Input: part model. Units: mm. Frame: model coordinates. Face numbers are marked on the shaded views. A direction names the side the tool comes from. Round coordinates to 2 decimals unless told otherwise and drop trailing zeros. Loops run counter-clockwise (first coordinate to the right, second up) from the corner with the lowest first, then second, coordinate; pieces in that order, holes last. Notation, with made-up numbers: (82, 65.25) - (112, 65.25) arc R6 cw to (112, 74.25) - close; hole circle Ø1 at (36.5, 53). An arc over 180 degrees is marked (long way). Use CSV: the item, a comma, the result in double quotes. Start each with the question number.
1. Cut plane A-A (y = -1.5). Return loops of the section in (x, z).
2. Cut plane B-B (x = 20). Return loops of the section in (y, z).
3. Access query for the marked faces 1 and 2. Directions: +Z, -Z, +X, -X, +Y, -Y. A direction counts if a zero-diameter tool reaches every point of the face in a straight line with its end or side. Return the directions, or none.
4. Cut plane C-C (y = -30). Return loops of the section in (x, z), and give its area (3 significant figures).
5. Pull-direction query (Y, two-part tool) for the marked faces 3, 4 and 5; classes: +Y half, -Y half, draft (parallel to the pull), parting line (faces both ways), or undercut.
6. Cut plane D-D (x = 6). Return loops of the section in (y, z).
7. Pin query (flat end, axial travel): P1, Ø0.6, axis at x = 4.5, y = 0.5, coming from the +Z side; P2, Ø0.6, axis at y = 0.5, z = 10, coming from the -X side; P3, Ø5.5, axis at y = -20, z = 10, coming from the +X side. Return the tip coordinate at first contact, or that it passes through.
8. Material intervals for probe 1 along Z at (x, y) = (2.1, -20); probe 2 along X at (y, z) = (-2.15, 10); probe 3 along Y at (x, z) = (0.9, 10), sorted ascending. Write a range as from..to.
```python
from build123d import *

# Parameters (mm, degrees)
BOSS_EXTRUDE1_DEPTH = 3.5
BOSS_EXTRUDE2_DEPTH = 16.5
SKETCH4_R           = 2.2
CUT_EXTRUDE1_DEPTH  = 53.773099208
SKETCH5_R           = 2.2
CUT_EXTRUDE2_DEPTH  = 53.773099208
BOSS_EXTRUDE5_DEPTH = 36
SKETCH7_W           = 15
SKETCH7_H           = 1.1
CUT_EXTRUDE3_DEPTH  = 53.496095093
BOSS_EXTRUDE6_REACH = 57.429
SKETCH9_W           = 1.1
SKETCH9_H           = 15
CUT_EXTRUDE4_DEPTH  = 53.496095093
BOSS_EXTRUDE7_DEPTH = 3.5
SKETCH11_R          = 1.6
CUT_EXTRUDE5_DEPTH  = 54.518688325


with BuildPart() as part:
    # Sketch1 → Boss-Extrude1 (new body)
    with BuildSketch(Plane.XY):
        Polygon((0, -36), (0, 0), (36, 0), (36, -3), (3, -36), align=None)
    extrude(amount=BOSS_EXTRUDE1_DEPTH)

    # Sketch2 → Boss-Extrude2 (add)
    with BuildSketch(Plane.XY.offset(3.5)):
        Polygon((0, -36), (0, 0), (36, 0), (36, -3), (3, -3), (3, -36), align=None)
    extrude(amount=BOSS_EXTRUDE2_DEPTH)

    # Sketch4 → Cut-Extrude1 (cut, through all)
    with BuildSketch(Plane.XZ.offset(3)):
        with Locations(Location((20, 10, 0), (0, 0, 270))):
            Circle(SKETCH4_R)
    extrude(amount=-CUT_EXTRUDE1_DEPTH, mode=Mode.SUBTRACT)

    # Sketch5 → Cut-Extrude2 (cut, through all)
    with BuildSketch(Plane(origin=(3, 0, 0), x_dir=(0, 0, -1), z_dir=(1, 0, 0))):
        with Locations((-10, -20)):
            Circle(SKETCH5_R)
    extrude(amount=-CUT_EXTRUDE2_DEPTH, mode=Mode.SUBTRACT)

    # Sketch6 → Boss-Extrude5 (add, through all)
    with BuildSketch(Plane(origin=(36, 0, 0), x_dir=(0, 0, -1), z_dir=(1, 0, 0))):
        Polygon((-12.8, 0), (-12.8, 1.1), (-9.6, 1.1), (-8.2, 0), align=None)
    extrude(amount=-BOSS_EXTRUDE5_DEPTH)

    # Sketch7 → Cut-Extrude3 (cut, through all)
    with BuildSketch(Plane.XY.offset(12.8)):
        with Locations((17.5, 0.55)):
            Rectangle(SKETCH7_W, SKETCH7_H)
    extrude(amount=-CUT_EXTRUDE3_DEPTH, mode=Mode.SUBTRACT)

    # Boss-Extrude6: up to this face of the body (flat: up to its plane)
    boss_extrude6_end = Plane(part.part.faces().sort_by_distance((0.411825206, 0, 16.4))[0])
    # Sketch8 → Boss-Extrude6 (add, up to the picked face)
    with BuildSketch(Plane.XZ.offset(36), mode=Mode.PRIVATE) as boss_extrude6_sk1:
        Polygon((0, 8.2), (0, 12.8), (-1.1, 12.8), (-1.1, 9.6), align=None)
    boss_extrude6_tool1 = split(extrude(boss_extrude6_sk1.sketch, amount=-BOSS_EXTRUDE6_REACH, mode=Mode.PRIVATE), bisect_by=boss_extrude6_end, keep=Keep.BOTH, mode=Mode.PRIVATE)
    add(boss_extrude6_tool1.solids().sort_by(Axis((-0.517094, -36, 10.82906), (0, 1, 0)))[0])

    # Sketch9 → Cut-Extrude4 (cut, through all)
    with BuildSketch(Plane.XY.offset(12.8)):
        with Locations((-0.55, -17.5)):
            Rectangle(SKETCH9_W, SKETCH9_H)
    extrude(amount=-CUT_EXTRUDE4_DEPTH, mode=Mode.SUBTRACT)

    # Sketch10 → Boss-Extrude7 (add)
    with BuildSketch(Plane.XY.offset(3.5)):
        Polygon((12.286392879, -26.713607121), (26.612382252, -12.387617748), (34.721916423, -18.238724953), (23.019702013, -34.457793296), align=None)
    extrude(amount=-BOSS_EXTRUDE7_DEPTH)

    # Sketch11 → Cut-Extrude5 (cut, through all)
    with BuildSketch(Plane.XY.offset(3.5)):
        with Locations((20.629708117, -20.629708117)):
            Circle(SKETCH11_R)
    extrude(amount=-CUT_EXTRUDE5_DEPTH, mode=Mode.SUBTRACT)


solid = part.part
```
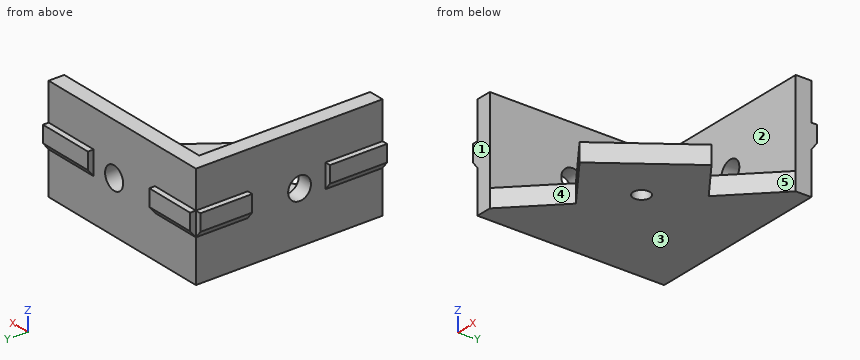
Established:
1,outline,"(-1.1, 9.6) - (0, 8.2) - (0, 0) - (36, 0) - (36, 20) - (0, 20) - (0, 12.8) - (-1.1, 12.8) - close; hole circle Ø4.4 at (20, 10)"
2,outline,"(-32.28, 0) - (-22.1, 0) - (-22.1, 3.5) - (-32.28, 3.5) - close; (-19.16, 0) - (0, 0) - (0, 7.8) - (-3, 7.8) - (-3, 3.5) - (-19.16, 3.5) - close; (-3, 12.2) - (0, 12.2) - (0, 20) - (-3, 20) - close"
3,face 1,"+Z, -Z, +X, -X, -Y"
3,face 2,"+Z, +X, -Y"
4,outline,"(-1.1, 9.6) - (0, 8.2) - (0, 0) - (9, 0) - (9, 3.5) - (3, 3.5) - (3, 20) - (0, 20) - (0, 12.8) - (-1.1, 12.8) - close; (16.84, 0) - (26.24, 0) - (26.24, 3.5) - (16.84, 3.5) - close"
4,area,"118 mm2"
5,face 3,"draft"
5,face 4,"-Y half"
5,face 5,"undercut"
6,outline,"(-33, 0) - (0, 0) - (0, 8.2) - (1.1, 9.6) - (1.1, 12.8) - (0, 12.8) - (0, 20) - (-3, 20) - (-3, 3.5) - (-33, 3.5) - close"
7,P1,"stops at z = 12.8"
7,P2,"stops at x = 0"
7,P3,"stops at x = 3"
8,probe 1,"z = 0..7.8, 12.2..20"
8,probe 2,"x = -1.1..17.8, 22.2..36"
8,probe 3,"y = -36..-22.2, -17.8..1.1"
